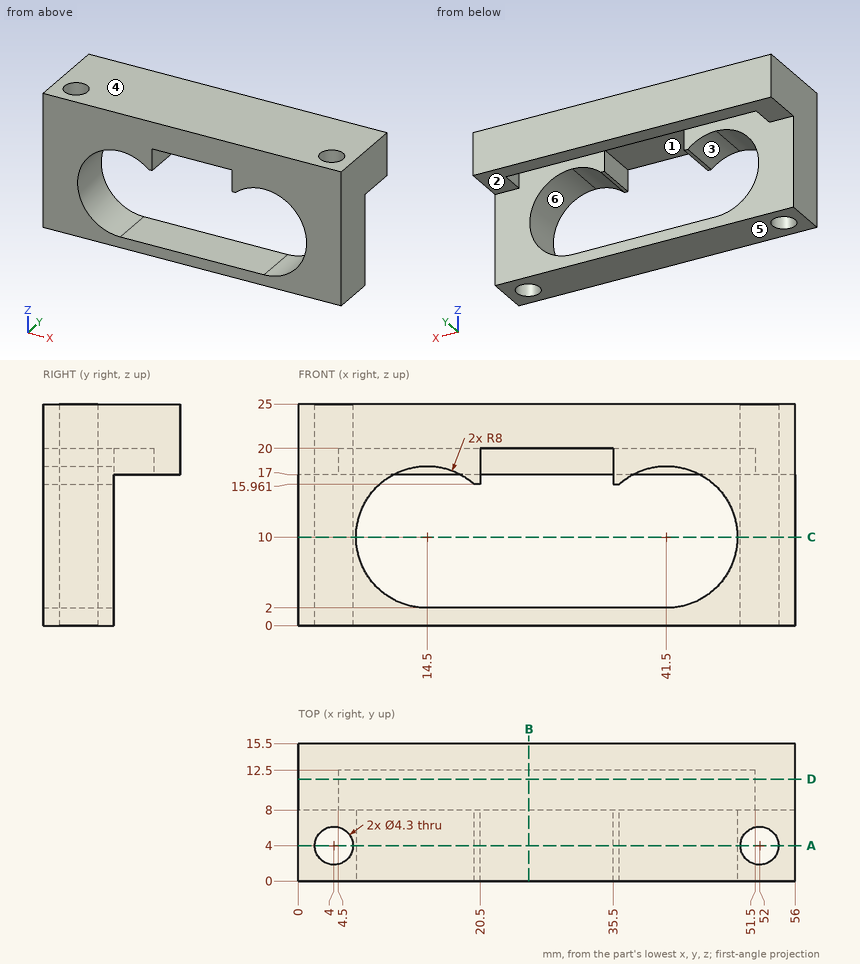
Can you work these out from the drawing? Everything is in mm from the part's minimum corner. A direction names the side the tool comes from. Round coordinates to 2 decimals unless told otherwise and drop trailing zeros. Order: outer loops, then holes, each group sorted by start corner. A loop starts at its lowest first (then second) coordinate and runs counter-clockwise, first axis right, second up.
(1) If I drill on L1, parallel to Z at x = 28, y = 1.75; L2, parallel to Y at x = 4, z = 10.5; L3, parallel to Z at x = 4, y = 9.5, over which ranges is the centre line in solid material (lowest first)?
Results are:
L1: z = 0 to 2, 20 to 25
L2: y = 0 to 1.85, 6.15 to 8
L3: z = 17 to 25
(2) We'd pull the mould along Z, two halves only. Please class the marked faces 4, 5 and 6: +Z half, -Z half, draft (parallel to the pull), parting line (faces both ways), or undercut.
Results are:
face 4: +Z half
face 5: -Z half
face 6: undercut
(3) If we section it at B-B (x = 26): Please give me the cut outline in (y, z), plus the area to 4 significant figures.
Results are:
outline: (0, 0) - (8, 0) - (8, 2) - (0, 2) - close; (0, 20) - (12.5, 20) - (12.5, 17) - (15.5, 17) - (15.5, 25) - (0, 25) - close
area: 102.5 mm2
(4) On a 3-axis mill with a long thin cutter (end or side, diameter ignored), from which of +Z, -Z, +X, -X, +Y, -Y can I reach the whole of each face in a straight line? I mean the marked faces 1, 2 and 3. Say none if no direction works.
Results are:
face 1: none
face 2: -Z, +X, -X, +Y
face 3: -Y
(5) If we section it at C-C (z = 10): Please give me the cut outline in (x, y).
Results are:
outline: (0, 0) - (6.5, 0) - (6.5, 8) - (0, 8) - close; (49.5, 0) - (56, 0) - (56, 8) - (49.5, 8) - close; hole circle Ø4.3 at (4, 4); hole circle Ø4.3 at (52, 4)
(6) If we section it at D-D (y = 11.5): Please give me the cut outline in (x, z).
Results are:
outline: (0, 17) - (4.5, 17) - (4.5, 20) - (51.5, 20) - (51.5, 17) - (56, 17) - (56, 25) - (0, 25) - close
(7) I'm going to push a flat-ended pin straight in: pin 1 (1.5 mm diameter, centred on x = 15, y = 13.5, fed in from -Z). Where does the tip first touch, or does it pass through?
Results are:
pin 1: stops at z = 17
(8) If we section it at A-A (y = 4): Please give me the cut outline in (x, z).
Results are:
outline: (0, 0) - (1.85, 0) - (1.85, 25) - (0, 25) - close; (6.15, 0) - (49.85, 0) - (49.85, 25) - (6.15, 25) - close; (54.15, 0) - (56, 0) - (56, 25) - (54.15, 25) - close; hole (14.5, 2) - (41.5, 2) arc R8 ccw to (41.5, 18) arc R8 ccw to (36.16, 15.96) - (35.5, 15.96) - (35.5, 20) - (20.5, 20) - (20.5, 15.96) - (19.84, 15.96) arc R8 ccw to (14.5, 18) arc R8 ccw to start
